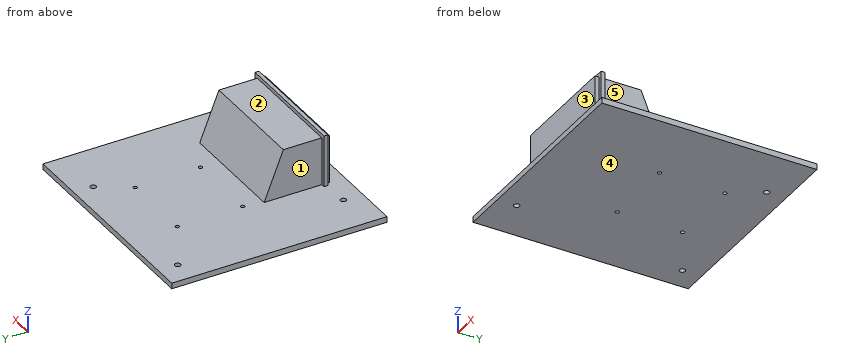
from build123d import *

# Parameters (mm, degrees)
CROQUIS1_W              = 116
CROQUIS1_H              = 112
SALIENTE_EXTRUIR1_DEPTH = 3
CROQUIS2_W              = 58
CROQUIS2_H              = 34
SALIENTE_EXTRUIR2_DEPTH = 25
CROQUIS3_W              = 62
CROQUIS3_H              = 27
SALIENTE_EXTRUIR3_DEPTH = 2
CORTAR_EXTRUIR1_DEPTH   = 116.117331449
CROQUIS5_R              = 1.5
CROQUIS5_R_2            = 1
CORTAR_EXTRUIR2_DEPTH   = 86.023526156


with BuildPart() as part:
    # Croquis1 → Saliente-Extruir1 (new body)
    with BuildSketch(Plane.XY):
        Rectangle(CROQUIS1_W, CROQUIS1_H)
    extrude(amount=SALIENTE_EXTRUIR1_DEPTH)

    # Croquis2 → Saliente-Extruir2 (add)
    with BuildSketch(Plane.XY.offset(3)):
        with Locations((9, -31)):
            Rectangle(CROQUIS2_W, CROQUIS2_H)
    extrude(amount=SALIENTE_EXTRUIR2_DEPTH)

    # Croquis3 → Saliente-Extruir3 (add)
    with BuildSketch(Plane(origin=(0, -46, 0), x_dir=(-1, 0, 0), z_dir=(0, -1, 0))):
        with Locations((-9, -16.5)):
            Rectangle(CROQUIS3_W, CROQUIS3_H)
    extrude(amount=-SALIENTE_EXTRUIR3_DEPTH)

    # Croquis4 → Cortar-Extruir1 (cut, through all)
    with BuildSketch(Plane(origin=(38, 0, 0), x_dir=(0, 0, -1), z_dir=(1, 0, 0))):
        Polygon((-3, -14), (-28, -24.000473789), (-28, -14), align=None)
    extrude(amount=-CORTAR_EXTRUIR1_DEPTH, mode=Mode.SUBTRACT)

    # Croquis5 → Cortar-Extruir2 (cut, through all)
    with BuildSketch(Plane.XY.offset(3)):
        with Locations((-36, -46)):
            Circle(CROQUIS5_R)
        with Locations((-46, 46)):
            Circle(CROQUIS5_R)
        with Locations((30, 46)):
            Circle(CROQUIS5_R)
        with Locations((20, 30)):
            Circle(CROQUIS5_R_2)
        with Locations((20, -4)):
            Circle(CROQUIS5_R_2)
        with Locations((-18, -4)):
            Circle(CROQUIS5_R_2)
        with Locations((-18, 30)):
            Circle(CROQUIS5_R_2)
    extrude(amount=-CORTAR_EXTRUIR2_DEPTH, mode=Mode.SUBTRACT)


solid = part.part
The listing builds one solid part. Answer for the finished solid, in the listing's coordinates (mm). Face numbers are marked on the shaded views. A direction names the side the tool comes from. Coordinates: 2 decimals unless noted, no trailing zeros. Order: outer loops, then holes, each group sorted by start corner. A loop starts at its lowest first (then second) coordinate and runs counter-clockwise, first axis right, second up. Notation, with made-up numbers: (57, 82.5) -> (115, 82.5) arc R16 cw to (115, 92.5) -> close; hole circle Ø5 at (49, 49.25). An arc over 180 degrees is marked (long way). Answer in a Markdown table with one row per item. Add a question column.
Item 1: Find the intervals of material crossed by L1, parallel to Y at x = -18, z = 1.35; L2, parallel to Y at x = 30, z = 1.7; L3, parallel to X at y = -39, z = 14.25, in increasing order. Write a range as from..to.
Item 2: Find section C-C (y = -41.5). Write down the section's boundary in (x, z).
Item 3: Find section A-A (x = 30). Write down the section's boundary in (y, z), then the cut area to 3 significant figures.
Item 4: Find section B-B (x = -46). Write down the section's boundary in (y, z).
Item 5: Find section D-D (x = 4). Write down the section's boundary in (y, z).
Item 6: Which of the six approach directions +Z, -Z, +X, -X, +Y, -Y give full straight-line access (tool end or side, diameter ignored) to the marked faces 1, 2, 3, 4 and 5?
Item 7: Each of these flat-tipped pins is pushed along its axis until it touches: P1, Ø2, axis at x = 17.5, z = 26.5, coming from the +Y side; P2, Ø1.5, axis at y = -18.5, z = 6, coming from the -X side; P3, Ø5, axis at x = 32, z = 23, coming from the +Y side. Where does it stop, or does it pass through?
Result set:
| question | item | result |
|---|---|---|
| 1 | L1 | y = -56..-5, -3..29, 31..56 |
| 1 | L2 | y = -56..44.5, 47.5..56 |
| 1 | L3 | x = -20..38 |
| 2 | outline | (-58, 0) -> (58, 0) -> (58, 3) -> (38, 3) -> (38, 28) -> (-20, 28) -> (-20, 3) -> (-58, 3) -> close |
| 3 | outline | (-56, 0) -> (44.5, 0) -> (44.5, 3) -> (-14, 3) -> (-24, 28) -> (-44, 28) -> (-44, 30) -> (-46, 30) -> (-46, 28) -> (-48, 28) -> (-48, 3) -> (-56, 3) -> close; (47.5, 0) -> (56, 0) -> (56, 3) -> (47.5, 3) -> close |
| 3 | area | 1,060 mm² |
| 4 | outline | (-56, 0) -> (44.5, 0) -> (44.5, 3) -> (-56, 3) -> close; (47.5, 0) -> (56, 0) -> (56, 3) -> (47.5, 3) -> close |
| 5 | outline | (-56, 0) -> (56, 0) -> (56, 3) -> (-14, 3) -> (-24, 28) -> (-44, 28) -> (-44, 30) -> (-46, 30) -> (-46, 28) -> (-48, 28) -> (-48, 3) -> (-56, 3) -> close |
| 6 | face 1 | +Z, -X, +Y |
| 6 | face 2 | +Z, +X, -X, +Y |
| 6 | face 3 | +Z, +X, -X, -Y |
| 6 | face 4 | -Z, +X, -X, +Y, -Y |
| 6 | face 5 | +Z, +X, +Y |
| 7 | P1 | stops at y = -23 |
| 7 | P2 | stops at x = -20 |
| 7 | P3 | stops at y = -21 |
